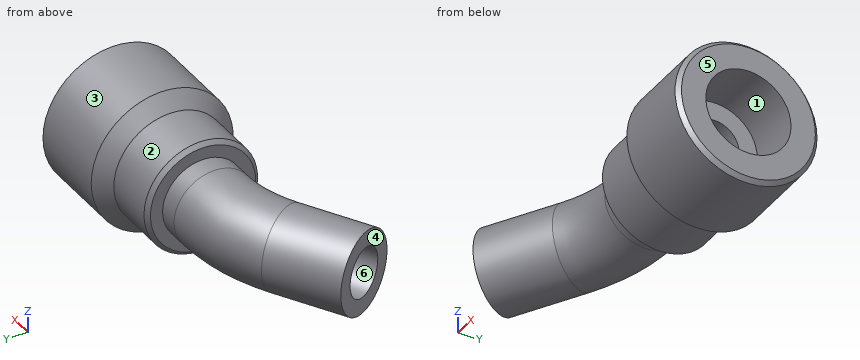
from build123d import *

# Parameters (mm, degrees)
CHAMFER1_SIZE = 1
SKETCH2_R     = 10
SKETCH2_R_2   = 6


with BuildPart() as part:
    # Sketch1 → Revolve1 (revolve)
    with BuildSketch(Plane.XY):
        Polygon((0, 10), (0, 14), (13.5, 14), (17, 17.5), (38, 17.5), (38, 10.5), (24, 10.5), (24, 6), (14.5, 6), (14.5, 10), align=None)
    revolve(axis=Axis((0, 0, 0), (1, 0, 0)))

    # Chamfer1
    chamfer1_edges = [part.edges().sort_by_distance(p)[0] for p in [
        (38, -17.5, 0),
        (0, -14, 0),
    ]]
    chamfer(chamfer1_edges, length=CHAMFER1_SIZE)

    # Sweep6: sweep along a path in Sketch3
    with BuildLine(Plane.XY) as sweep6_path:
        Line((14.5, 0), (-4.782032303, 0))
        ThreePointArc((-4.782032303, 0), (-15.134794107, -1.362966948), (-24.782032303, -5.358983849))
        Line((-24.782032303, -5.358983849), (-41.480762114, -15))
    # Sketch2 → Sweep6 (sweep)
    with BuildSketch(Plane.ZY.offset(-14.5)):
        Circle(SKETCH2_R)
        Circle(SKETCH2_R_2, mode=Mode.SUBTRACT)
    sweep(path=sweep6_path.line)


solid = part.part
Input: part model. Units: mm. Frame: model coordinates. Face numbers are marked on the shaded views. A direction names the side the tool comes from. Coordinates: 2 decimals unless noted, no trailing zeros. Order: outer loops, then holes, each group sorted by start corner. A loop starts at its lowest first (then second) coordinate and runs counter-clockwise, first axis right, second up. Notation, with made-up numbers: M -18.5,38.25 L 6.5,38.25 A8 ccw 6.5,47.25 Z; hole C 67.25,58.5 d7. An arc over 180 degrees is marked long. Answer in a Markdown table with one row per item.
(1) Section query B-B, the plane x = 7.5. Output: boundary loops of the cut face in (y, z).
Numbers:
| item | result |
|---|---|
| outline | C 0,0 d28; hole C 0,0 d12 |
(2) Contact query for flat-ended pins moving along their axis: pin 1 Ø10 at (x, z) = (-17.5, 4) entering from -Y; pin 2 Ø10 at (x, y) = (12.5, -16) entering from +Z; pin 3 Ø5 at (y, z) = (-8.5, -5) entering from -X; pin 4 Ø8 at (x, y) = (-9, -17.5) entering from +Z. Output: stop coordinate, or through.
Numbers:
| item | result |
|---|---|
| pin 1 | stops at y = -15.11 |
| pin 2 | stops at z = 10.95 |
| pin 3 | stops at x = -46.22 |
| pin 4 | passes through |
(3) Material intervals for line 1 (Z direction, x = 30.5, y = 0); line 2 (Z direction, x = 20.5, y = 0); line 3 (Y direction, x = 26, z = 8), sorted ascending. Write a range as [from, to].
Numbers:
| item | result |
|---|---|
| line 1 | z = [-17.5, -10.5], [10.5, 17.5] |
| line 2 | z = [-17.5, -6], [6, 17.5] |
| line 3 | y = [-15.56, -6.8], [6.8, 15.56] |
(4) Draft query along Y for the marked faces 3, 4, 5 and 6. Return one class per face: pulls with the +Y half, pulls with the -Y half, needs draft (parallel to the pull), parting line crosses it, or undercut.
Numbers:
| item | result |
|---|---|
| face 3 | parting line crosses it |
| face 4 | pulls with the -Y half |
| face 5 | needs draft |
| face 6 | undercut |
(5) Access query for the marked faces 1 and 2. Directions: +Z, -Z, +X, -X, +Y, -Y. A direction counts if a zero-diameter tool reaches every point of the face in a straight line with its end or side. Return the directions, or none.
Numbers:
| item | result |
|---|---|
| face 1 | +X |
| face 2 | none |
